Design review of the part built by this model. Coordinates are the model's own, in mm. A direction names the side the tool comes from. Coordinates: 2 decimals unless noted, no trailing zeros. Loops run counter-clockwise (first coordinate to the right, second up) from the corner with the lowest first, then second, coordinate; pieces in that order, holes last. Notation, with made-up numbers: (-23, -8) -> (-8, -8) arc R20 ccw to (-8, 9) -> close; hole circle Ø4 at (12, 83.5). An arc over 180 degrees is marked (long way). Answer in a Markdown table with one row per item.
```python
from build123d import *

# Parameters (mm, degrees)
SKETCH039_R      = 2.5
PAD023_DEPTH     = 58
POCKET003_DEPTH  = 18
CHAMFER002_SIZE2 = 0.4
CHAMFER002_SIZE  = 0.8


with BuildPart() as part:
    # Sketch039 → Pad023 (new body)
    with BuildSketch(Plane.XY):
        Circle(SKETCH039_R)
    extrude(amount=PAD023_DEPTH)

    # Sketch040 (on Face3 of Pad023) → Pocket003 (cut)
    with BuildSketch(Plane.XY.offset(58)):
        with BuildLine():
            ThreePointArc((2, -1.5), (2.5, 0), (2, 1.5))
            Line((2, 1.5), (2, -1.5))
        make_face()
    extrude(amount=-POCKET003_DEPTH, mode=Mode.SUBTRACT)

    # Chamfer002
    chamfer002_edges = [part.edges().sort_by_distance(p)[0] for p in [
        (-2.5, 0, 58),
        (-2.5, 0, 0),
    ]]
    chamfer002_side = part.faces().sort_by_distance((-2.5, 0, 29))[0]
    chamfer(chamfer002_edges, length=CHAMFER002_SIZE, length2=CHAMFER002_SIZE2, reference=chamfer002_side)


with BuildPart() as part_1:
    # Body012 placement: moved
    add(part.part.moved(Location((0, 0, 2.8))))


solid = part_1.part
```
(1) Take a section at B-B on z = 21. Give the boundary of the cut face in (x, y), and give its area (3 significant figures).
Evaluation:
| item | result |
|---|---|
| outline | circle Ø5 at (0, 0) |
| area | 19.6 mm² |
(2) Take a section at C-C on z = 47.5. Give the boundary of the cut face in (x, y).
Evaluation:
| item | result |
|---|---|
| outline | (2, -1.5) -> (2, 1.5) arc R2.5 ccw (long way) to start |
(3) Tool access review of faces 1 (the flat face through (2, 0, 52)), 2 (the cylindrical face through (-2.5, 0.1, 31.4)): name each direction out of +Z, -Z, +X, -X, +Y, -Y from which nothing blocks a thin tool from reaching the whole face with its end or side.
Evaluation:
| item | result |
|---|---|
| face 1 | +Z, +X, +Y, -Y |
| face 2 | +Z, -Z |
(4) Take a section at A-A on y = 0. Give the boundary of the cut face in (x, z), and give its area (3 significant figures).
Evaluation:
| item | result |
|---|---|
| outline | (-2.5, 3.6) -> (-2.1, 2.8) -> (2.1, 2.8) -> (2.5, 3.6) -> (2.5, 42.8) -> (2, 42.8) -> (2, 60.8) -> (-2.1, 60.8) -> (-2.5, 60) -> close |
| area | 281 mm² |
(5) To check wall thickness, follow probe 1 along Y at (x, z) = (0.1, 30); probe 2 along Y at (x, z) = (2, 32); probe 3 along X at (y, z) = (0.2, 12). State the ranges of each line that lie inside material, in increasing order.
Evaluation:
| item | result |
|---|---|
| probe 1 | y = -2.5 to 2.5 |
| probe 2 | y = -1.5 to 1.5 |
| probe 3 | x = -2.49 to 2.49 |
(6) For pin 1 (0.5 mm diameter, centred on x = 2.5, y = 0, fed in from +Z); pin 2 (1.5 mm diameter, centred on x = -1.5, z = 37, fed in from -Y); pin 3 (2.5 mm diameter, centred on y = -0.5, z = 49, fed in from +X), all flat-tipped, find the tip position at first contact; note any pin that passes through.
Evaluation:
| item | result |
|---|---|
| pin 1 | stops at z = 42.8 |
| pin 2 | stops at y = -2.38 |
| pin 3 | stops at x = 2 |
